from build123d import *

# Parameters (mm, degrees)
F0_W        = 50
F0_H        = 15
F1_DEPTH    = 15
F2_R        = 7.49999
F3_R        = 3.5
F4_DEPTH    = 25
F6_DEPTH    = 30
F7_SIZE     = 2
F8_T1_DEPTH = 36.7168298797
F8_T3_DEPTH = 36.7168298797


# Not quite as in the source:
# - a fillet or chamfer that OpenCascade refuses, or shapes differently, is made with other operations: its cross-section is extruded or revolved along the edge and cut away or added
# - a fillet or chamfer is up to 0.001 mm smaller than in the source, because OpenCascade refuses the exact size


with BuildPart() as f1:
    # F0 (on Top) → F1 (new body)
    with BuildSketch(Plane.XY):
        with Locations((-34.3210311607, 15.3476024792)):
            Rectangle(F0_W, F0_H)
    extrude(amount=F1_DEPTH)

    # F2 (radius 7.5 in the source; OpenCascade refuses exactly that, so slightly less here)
    f2_edges = [f1.edges().sort_by_distance(p)[0] for p in [
        (-59.321031, 22.847602, 7.5),
        (-59.321031, 7.847602, 7.5),
    ]]
    fillet(f2_edges, radius=F2_R)

    # F3 (on face) → F4 (cut)
    with BuildSketch(Plane.XY.offset(15)):
        with Locations((-51.8210311607, 15.3476024792)):
            Circle(F3_R)
    extrude(amount=-F4_DEPTH, mode=Mode.SUBTRACT)

    # F5 (on face) → F6 (cut)
    with BuildSketch(Plane.YZ.offset(-9.3210311607)):
        with BuildLine():
            ThreePointArc((18.8476024792, 7.5), (15.3476024792, 11), (11.8476024792, 7.5))
            ThreePointArc((11.8476024792, 7.5), (15.3476024792, 4), (18.8476024792, 7.5))
        make_face()
    extrude(amount=-F6_DEPTH, mode=Mode.SUBTRACT)

    # F7
    f7_edges = [f1.edges().sort_by_distance(p)[0] for p in [
        (-30.571036, 7.847602, 15),
        (-30.571036, 7.847602, 0),
    ]]
    chamfer(f7_edges, length=F7_SIZE)

    # F8: chamfer of 5 on 4 edges, made by hand

    # F8_s2 → F8_t1 (cut)
    with BuildSketch(Plane.XZ.offset(-33.706017419)):
        Polygon((-9.3210311607, 10), (-14.3210311607, 15), (-9.3210311607, 15), align=None)
        Polygon((-9.3210311607, 5), (-14.3210311607, 0), (-9.3210311607, 0), align=None)
    extrude(amount=F8_T1_DEPTH, mode=Mode.SUBTRACT)

    # F8_s4 → F8_t3 (cut)
    with BuildSketch(Plane.XY.offset(-10.8584149398)):
        Polygon((-9.3210311607, 12.8476024792), (-14.3210311607, 7.8476024792), (-9.3210311607, 7.8476024792), align=None)
        Polygon((-14.3210311607, 22.8476024792), (-9.3210311607, 17.8476024792), (-9.3210311607, 22.8476024792), align=None)
    extrude(amount=F8_T3_DEPTH, mode=Mode.SUBTRACT)


solid = f1.part
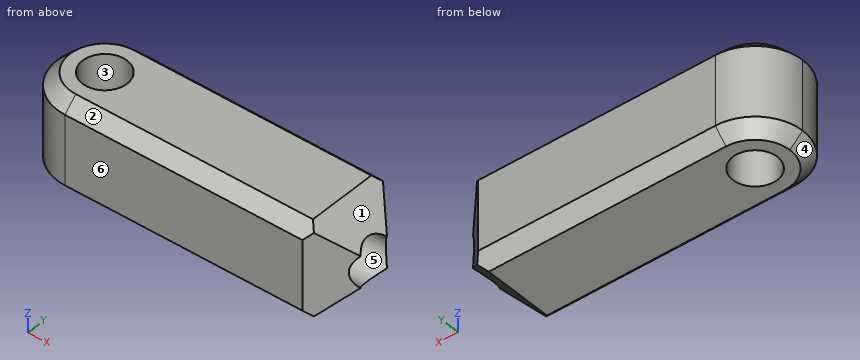
The listing builds one solid part. Answer for the finished solid, in the listing's coordinates (mm). Face numbers are marked on the shaded views. A direction names the side the tool comes from. Give positions to 0.01 mm unless a question says otherwise; leave off trailing zeros. Order: outer loops, then holes, each group sorted by start corner. A loop starts at its lowest first (then second) coordinate and runs counter-clockwise, first axis right, second up. Notation, with made-up numbers: (5.5, -0.5) - (55.5, -0.5) arc R12 ccw to (55.5, 7.5) - close; hole circle Ø5 at (77.5, 7). An arc over 180 degrees is marked (long way). One line per item, written item: value. Start each with the question number.
1) A cutting plane is placed at A-A on x = -33.5. Give the vertices of the cut face in (y, z).
2) Find the intervals of material crossed by L1, parallel to Y at x = -26, z = 7.5; L2, parallel to Y at x = -29, z = 7.75; L3, parallel to X at y = 13.75, z = 5.5, in increasing order.
3) A tool of negligible diameter and unlimited length cuts with its end or side. For the marked faces 5 and 6, from which of +Z, -Z, +X, -X, +Y, -Y can it reach the whole face along a straight path? Write none if from no direction.
4) Given pin 1 Ø4 at (y, z) = (11, 2) entering from -X; pin 2 Ø3.5 at (y, z) = (16, 8.5) entering from +X; pin 3 Ø1.5 at (y, z) = (9.5, 13.5) entering from -X, each flat-ended and moving along its own axis, determine where each tip first touches the part or whether it passes through.
5) A cutting plane is placed at B-B on x = -47. Give the vertices of the cut face in (y, z).
6) The mould has two halves that part along X. Classify the marked faces 1, 2, 3 and 4: released by +X, released by -X, zero draft, split by the parting line, or undercut.
Answer sheet:
1. outline: (7.85, 2) - (9.85, 0) - (20.85, 0) - (22.85, 2) - (22.85, 13) - (20.85, 15) - (9.85, 15) - (7.85, 13) - close; hole circle Ø7 at (15.35, 7.5)
2. L1: y = 7.85 to 11.85, 18.85 to 22.85
2. L2: y = 7.85 to 11.86, 18.84 to 22.85
2. L3: x = -59.15 to -54.94, -48.71 to -39.32
3. face 5: +X
3. face 6: +Z, -Z, +X, -X, -Y
4. pin 1: stops at x = -58.94
4. pin 2: stops at x = -39.32
4. pin 3: stops at x = -57.14
5. outline: (7.85, 2) - (9.85, 0) - (20.85, 0) - (22.85, 2) - (22.85, 13) - (20.85, 15) - (9.85, 15) - (7.85, 13) - close
6. face 1: released by +X
6. face 2: zero draft
6. face 3: undercut
6. face 4: released by -X
